Could you check a few things on this model? Use its own coordinates, in mm. A direction names the side the tool comes from. Round coordinates to 2 decimals unless told otherwise and drop trailing zeros. Loops run counter-clockwise (first coordinate to the right, second up) from the corner with the lowest first, then second, coordinate; pieces in that order, holes last. Notation, with made-up numbers: (38, 36) -> (85, 36) arc R22 cw to (85, 47) -> close; hole circle Ø1 at (60, 14.5). An arc over 180 degrees is marked (long way). Put each result on its own line as item: value. Start each with the question number.
1. Imagine slicing it at A-A, the plane z = 4. Please give me the cut outline in (x, y), and give its area (3 significant figures).
2. I need wall thicknesses on line 1 (Y direction, x = 72.5, z = -28.5); line 2 (Y direction, x = 9.5, z = -1); line 3 (Y direction, x = -82.5, z = 19.5). Which ranges of each line are inside material? Lowest first, please. Write a range as [from, to].
3. Imagine slicing it at B-B, the plane x = -71.5. Please give me the cut outline in (y, z).
4. I'm going to push flat-ended pins straight in: P1, Ø6, axis at y = 46, z = 23.5, coming from the +X side; P2, Ø10, axis at y = 10.5, z = 4.5, coming from the +X side; P3, Ø10, axis at x = 31, z = 12.5, coming from the +Y side. Where does each tip first touch, or does it pass through?
5. If we mould it in two halves opening along Y, with no side actions, what happens to faces 5 (the flat face through (-67, -58.505, 1)), 6 (the flat face through (-74, 83.382, 1)), 7 (the flat face through (-32.777, -42.73, -18.783))? For each: pulls with the +Y half, pulls with the -Y half, needs draft (parallel to the pull), parting line crosses it, or undercut.
6. Which directions (+Z, -Z, +X, -X, +Y, -Y) give clear straight access to the entire face, cutting with the end or side of a thin tool? Please do faces 1 (the flat face through (91.837, 60, 1)), 2 (the flat face through (0, -34.801, -19)), 3 (the flat face through (11, 57.158, 1)), 4 (the flat face through (-84.54, -29, 22)).
7. Imagine slicing it at C-C, the plane y = 73.5. Please give me the cut outline in (x, z).
8. Imagine slicing it at D-D, the plane y = 16. Please give me the cut outline in (x, z).
```python
from build123d import *

# Parameters (mm, degrees)
F1_DEPTH = 38.1
F2_DEPTH = 6.35


with BuildPart() as f1:
    # F0 (on Top) → F1 (new body, symmetric)
    with BuildSketch(Plane.XY):
        Polygon((-83.179305, 18.750736), (-83.179305, 6.050736), (-92.159561, -2.92952), (-92.159561, -58.50472), (-42.019961, -58.50472), (-19.05, -42.42098), (-2.855429, -42.42098), (-2.855429, -37.99941), (2.855429, -37.99941), (2.855429, -42.42098), (19.05, -42.42098), (42.019961, -58.50472), (92.286561, -58.50472), (92.286561, -12.27672), (81.638513, 2.930269), (81.638513, 23.250269), (91.836702, 37.814792), (91.836702, 83.382392), (56.403702, 83.382392), (18.95207, 57.158478), (3.221597, 57.158478), (3.221597, 53.102199), (-3.36058, 53.102199), (-3.36058, 57.158478), (-19.14793, 57.158478), (-56.599561, 83.382392), (-92.159561, 83.382392), (-92.159561, 27.730992), align=None)
        Polygon((-84.539561, 30.8873), (-84.539561, 75.762392), (-59.002138, 75.762392), (-21.550506, 49.538478), (21.354647, 49.538478), (58.806279, 75.762392), (84.216702, 75.762392), (84.216702, 40.217369), (74.018513, 25.652846), (74.018513, 0.527692), (84.666561, -14.679297), (84.666561, -50.88472), (44.422538, -50.88472), (21.452577, -34.80098), (-21.452577, -34.80098), (-44.422538, -50.88472), (-84.539561, -50.88472), (-84.539561, -6.085827), (-75.559305, 2.894429), (-75.559305, 21.907044), align=None, mode=Mode.SUBTRACT)
    extrude(amount=F1_DEPTH, both=True)

    # F0 (on Top) → F2 (join)
    with BuildSketch(Plane.XY):
        Polygon((-59.002138, 75.762392), (-84.539561, 75.762392), (-84.539561, 30.8873), (-75.559305, 21.907044), (-75.559305, 2.894429), (-84.539561, -6.085827), (-84.539561, -50.88472), (-44.422538, -50.88472), (-21.452577, -34.80098), (21.452577, -34.80098), (44.422538, -50.88472), (84.666561, -50.88472), (84.666561, -14.679297), (74.018513, 0.527692), (74.018513, 25.652846), (84.216702, 40.217369), (84.216702, 75.762392), (58.806279, 75.762392), (21.354647, 49.538478), (-21.550506, 49.538478), align=None)
    extrude(amount=F2_DEPTH)


solid = f1.part
```
Entries:
1. outline: (-92.16, -58.5) -> (-42.02, -58.5) -> (-19.05, -42.42) -> (-2.86, -42.42) -> (-2.86, -38) -> (2.86, -38) -> (2.86, -42.42) -> (19.05, -42.42) -> (42.02, -58.5) -> (92.29, -58.5) -> (92.29, -12.28) -> (81.64, 2.93) -> (81.64, 23.25) -> (91.84, 37.81) -> (91.84, 83.38) -> (56.4, 83.38) -> (18.95, 57.16) -> (3.22, 57.16) -> (3.22, 53.1) -> (-3.36, 53.1) -> (-3.36, 57.16) -> (-19.15, 57.16) -> (-56.6, 83.38) -> (-92.16, 83.38) -> (-92.16, 27.73) -> (-83.18, 18.75) -> (-83.18, 6.05) -> (-92.16, -2.93) -> close
1. area: 22,600 mm^2
2. line 1: [-58.5, -50.88], [75.76, 83.38]
2. line 2: [-42.42, -34.8], [49.54, 57.16]
2. line 3: [-58.5, -50.88], [-4.05, 28.85], [75.76, 83.38]
3. outline: (-58.5, -38.1) -> (-50.88, -38.1) -> (-50.88, 0) -> (75.76, 0) -> (75.76, -38.1) -> (83.38, -38.1) -> (83.38, 38.1) -> (75.76, 38.1) -> (75.76, 6.35) -> (-50.88, 6.35) -> (-50.88, 38.1) -> (-58.5, 38.1) -> close
4. P1: x = 91.84
4. P2: x = 81.64
4. P3: y = 69.1
5. face 5: pulls with the -Y half
5. face 6: pulls with the +Y half
5. face 7: undercut
6. face 1: +Z, -Z, +X, +Y
6. face 2: -Z
6. face 3: +Z, -Z, +Y
6. face 4: +Z
7. outline: (-92.16, -38.1) -> (-84.54, -38.1) -> (-84.54, 0) -> (-55.77, 0) -> (-55.77, -38.1) -> (-42.49, -38.1) -> (-42.49, 38.1) -> (-55.77, 38.1) -> (-55.77, 6.35) -> (-84.54, 6.35) -> (-84.54, 38.1) -> (-92.16, 38.1) -> close; (42.29, -38.1) -> (55.58, -38.1) -> (55.58, 0) -> (84.22, 0) -> (84.22, -38.1) -> (91.84, -38.1) -> (91.84, 38.1) -> (84.22, 38.1) -> (84.22, 6.35) -> (55.58, 6.35) -> (55.58, 38.1) -> (42.29, 38.1) -> close
8. outline: (-83.18, -38.1) -> (-75.56, -38.1) -> (-75.56, 0) -> (74.02, 0) -> (74.02, -38.1) -> (81.64, -38.1) -> (81.64, 38.1) -> (74.02, 38.1) -> (74.02, 6.35) -> (-75.56, 6.35) -> (-75.56, 38.1) -> (-83.18, 38.1) -> close
